from build123d import *

# Parameters (mm, degrees)
F0_W     = 25.4
F0_H     = 38.1
F1_DEPTH = 4.7625
F2_W     = 25.4
F2_H     = 38.1
F2_R     = 3.96875
F3_DEPTH = 2.38125


# Not quite as in the source:
# - a length typed as a fraction of an inch, garbled in the dataset ("3 / 203.2 mm" for 3/8 in), is restored


with BuildPart() as f1:
    # F0 (on Top) → F1 (new body)
    with BuildSketch(Plane.XY):
        with Locations((0, -6.35)):
            Rectangle(F0_W, F0_H)
        with BuildLine():
            ThreePointArc((-8.73125, 0), (0, 8.73125), (8.73125, 0))
            Line((8.73125, 0), (8.73125, -19.05))
            Line((8.73125, -19.05), (-8.73125, -19.05))
            Line((-8.73125, -19.05), (-8.73125, 0))
        make_face(mode=Mode.SUBTRACT)
    extrude(amount=F1_DEPTH)

    # F2 (on face) → F3 (join)
    with BuildSketch(Plane.XY.offset(4.7625)):
        with Locations((0, -6.35)):
            Rectangle(F2_W, F2_H)
        Circle(F2_R, mode=Mode.SUBTRACT)
    extrude(amount=F3_DEPTH)


solid = f1.part
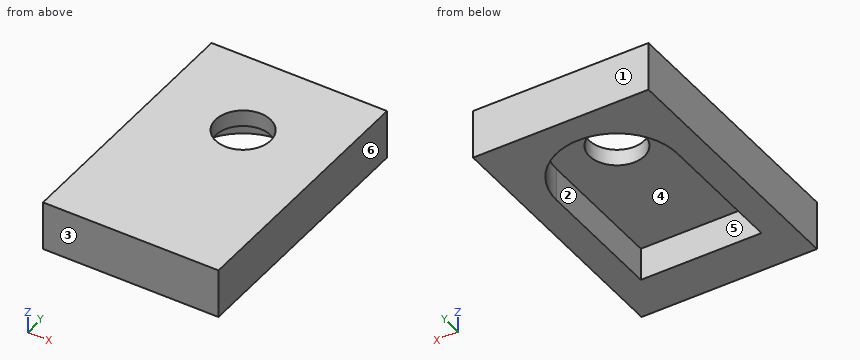
Geometry check sheet. Reference: the model listing, model coordinates, mm. Face numbers are marked on the shaded views. A direction names the side the tool comes from. Give positions to 0.01 mm unless a question says otherwise; leave off trailing zeros. Loops run counter-clockwise (first coordinate to the right, second up) from the corner with the lowest first, then second, coordinate; pieces in that order, holes last. Notation, with made-up numbers: M -13.75,-29.5 L 14.25,-29.5 A10 cw 14.25,-15.5 Z; hole C 62.5,65 d8. An arc over 180 degrees is marked long. Write each question's results on one line, items separated by ' | '.
1) Gauge pin test, flat end, axial feed: pin 1 (7 mm diameter, centred on x = 0, y = 0, fed in from -Z). Record the tip position at first contact, or that the pin passes through.
Answers follow:
pin 1: through
2) Tool access check on the marked faces 1 and 2. Record the directions out of +Z, -Z, +X, -X, +Y, -Y that give a thin tool (end or side, any length) a straight path to the whole face; none if there is none.
Answers follow:
face 1: +Z, -Z, +X, -X, +Y | face 2: -Z
3) Section check D-D, the plane y = -13.5. Record the boundary of the cut face in (x, z).
Answers follow:
outline: M -12.7,0 L -8.73,0 L -8.73,4.76 L 8.73,4.76 L 8.73,0 L 12.7,0 L 12.7,7.14 L -12.7,7.14 Z
4) Section check A-A, the plane x = 0. Record the boundary of the cut face in (y, z), plus the area to 3 significant figures.
Answers follow:
outline: M -25.4,0 L -19.05,0 L -19.05,4.76 L -3.97,4.76 L -3.97,7.14 L -25.4,7.14 Z; M 3.97,4.76 L 8.73,4.76 L 8.73,0 L 12.7,0 L 12.7,7.14 L 3.97,7.14 Z | area: 121 mm2
5) Thickness scan on line 1 (X direction, y = -6.5, z = 0.75); line 2 (Y direction, x = 0, z = 5.5); line 3 (Y direction, x = -3, z = 5). Record the ranges inside material, lowest first.
Answers follow:
line 1: -12.7 to -8.73, 8.73 to 12.7 | line 2: -25.4 to -3.97, 3.97 to 12.7 | line 3: -25.4 to -2.6, 2.6 to 12.7
6) Release check for a two-part mould opening along X. For the marked faces 3, 4, 5 and 6 record: +X half, -X half, draft (parallel to the pull), parting line (faces both ways), or undercut.
Answers follow:
face 3: draft | face 4: undercut | face 5: undercut | face 6: +X half
7) Section check C-C, the plane y = 2. Record the boundary of the cut face in (x, z), plus the area to 3 significant figures.
Answers follow:
outline: M -12.7,0 L -8.5,0 L -8.5,4.76 L -3.43,4.76 L -3.43,7.14 L -12.7,7.14 Z; M 3.43,4.76 L 8.5,4.76 L 8.5,0 L 12.7,0 L 12.7,7.14 L 3.43,7.14 Z | area: 84.2 mm2
8) Section check B-B, the plane z = 4. Record the boundary of the cut face in (x, y), plus the area to 3 significant figures.
Answers follow:
outline: M -12.7,-25.4 L 12.7,-25.4 L 12.7,12.7 L -12.7,12.7 Z; hole M -8.73,-19.05 L 8.73,-19.05 L 8.73,0 A8.73 ccw -8.73,0 Z | area: 515 mm2
